Work out the finished part from the listing and answer in its coordinate system (mm). A direction names the side the tool comes from. Give positions to 0.01 mm unless a question says otherwise; leave off trailing zeros. Write each loop counter-clockwise with the first axis right and the second up, starting at its lowest first coordinate (ties: lowest second). Pieces come first, ordered by that corner, then holes. Notation, with made-up numbers: (15, 55.5) -> (22, 55.5) arc R31 ccw to (22, 82.5) -> close; hole circle Ø10 at (-30.75, -22). An arc over 180 degrees is marked (long way). Write item = value, one per line. Start each with the question number.
Autodesk Inventor part; units mm, degrees
ref_plane "YZ Plane" through (0, 0, 0) normal (1, 0, 0) x (0, 1, 0)
ref_plane "XZ Plane" through (0, 0, 0) normal (0, 1, 0) x (-1, 0, 0)
ref_plane "XY Plane" through (0, 0, 0) normal (0, 0, 1) x (1, 0, 0)
sketch "Sketch1" plane through (0, 0, 0) normal (0, 0, 1) x (1, 0, 0)
  circle A0 centre (0, 0) radius 1.778
  circle A1 centre (0, 0) radius 32.512
  circle A2 centre (0, 0) radius 26.162
  circle A3 centre (0, 0) radius 6.858
  line L0 (-3.048, 6.1434) -> (-6.8485, 25.2497)
  line L1 (3.048, 6.1434) -> (6.8485, 25.2497)
  arc A4 (6.8485, 25.2497) -> (-6.8485, 25.2497) centre (0, 0) ccw construction
  line L2 (-6.7846, -1.0004) -> (-26.1302, 1.2893)
  circle A5 centre (0, 0) radius 26.162
  line L3 (-4.9009, 4.7972) -> (-21.8976, 14.3159)
  circle A6 centre (0, 0) radius 6.858
  line L4 (-1.1451, -6.7617) -> (-9.3009, -24.4529)
  circle A7 centre (0, 0) radius 26.162
  line L5 (-6.0769, -3.1786) -> (-20.3819, -16.402)
  circle A8 centre (0, 0) radius 6.858
  line L6 (6.0769, -3.1786) -> (20.3819, -16.402)
  circle A9 centre (0, 0) radius 26.162
  line L7 (1.1451, -6.7617) -> (9.3009, -24.4529)
  circle A10 centre (0, 0) radius 6.858
  line L8 (4.9009, 4.7972) -> (21.8976, 14.3159)
  circle A11 centre (0, 0) radius 26.162
  line L9 (6.7846, -1.0004) -> (26.1302, 1.2893)
  circle A12 centre (0, 0) radius 6.858
  dimension "d1" = 65.024
  dimension "d2" = 3.556
  dimension "d3" = 13.716
  dimension "d4" = 6.35
  dimension "d5" = 22.5
  dimension "d7" = 3.048
  dimension "d10" = 360
extrude "Extrusion1" add sketch "Sketch1" along normal blind 26.924 contours A1 | A3
extrude "Extrusion2" add sketch "Sketch1" along normal blind 21.59 contours A0
extrude "Extrusion3" add sketch "Sketch1" along normal blind 5.334 contours L9 A3 L8 A2 | A2 L7 A3 L6 | L1 A3 L0 A2 | A2 L5 A3 L4 | L3 A3 L2 A2
fillet "Fillet1" radius 3.175 2 edges at (-32.512, 0, 26.924) (-32.512, 0, 0)
properties part number "OGWheel" material "ABS Plastic"
(1) Find the intervals of material crossed by line 1 along Y through (x, z) = (1, 9.5); line 2 along Y through (x, z) = (0, 13); line 3 along Y through (x, z) = (0, 25.6), in increasing order.
(2) For faces 1 (the flat face through (5.166, -15.483, 2.63)), 2 (the flat face through (1.4, -1.4, 26.924)), 3 (the cylindrical face through (6.54, -2.06, 16.27)), determine the directions among +Z, -Z, +X, -X, +Y, -Y from which every point of the face is accessible in a straight line to the end or side of a thin tool.
(3) Each of these flat-tipped pins is pushed along its axis until it touches: pin 1 (7.5 mm diameter, centred on x = 19.5, y = 5.5, fed in from +Z); pin 2 (10 mm diameter, centred on y = -16.5, z = 13.5, fed in from -X); pin 3 (2 mm diameter, centred on x = -22, y = 24, fed in from +Z). Where does it stop, or does it pass through?
(4) A cutting plane is placed at A-A, the plane x = 0. Write down the section's boundary in (y, z) (3 decimals).
(5) A cutting plane is placed at D-D, the plane x = -12.5. State how many separate pieces and enclosed holes the cut face has, then the cut area to 3 significant figures.
(6) A cutting plane is placed at C-C, the plane y = 0. Write down the section's boundary in (x, z) (3 decimals).
(7) A cutting plane is placed at B-B, the plane z = 16.5. Write down the section's boundary in (x, y), then the cut area to 3 significant figures.
(8) Determine the mould class of faces 4 (the flat face through (-4.92, 15.56, 2.63)), 5 (the flat face through (-26.2, -4.2, 26.924)) for opening direction Y: pulls with the +Y half, pulls with the -Y half, needs draft (parallel to the pull), parting line crosses it, or undercut.
Results list:
q1.line_1 = -32.5 to -26.14, -6.78 to 6.78, 26.14 to 32.5
q1.line_2 = -32.51 to -26.16, -6.86 to 6.86, 26.16 to 32.51
q1.line_3 = -31.92 to -26.16, -6.86 to -1.78, 1.78 to 6.86, 26.16 to 31.92
q2.face_1 = +Z, -Z
q2.face_2 = +Z, +X, -X, +Y, -Y
q2.face_3 = +Z
q3.pin_1 = 5.33
q3.pin_2 = -30.41
q3.pin_3 = 26.02
q4.outline = (-32.512, 3.175) arc R3.175 ccw to (-29.337, 0) -> (-26.162, 0) -> (-26.162, 26.924) -> (-29.337, 26.924) arc R3.175 ccw to (-32.512, 23.749) -> close; (-6.858, 0) -> (29.337, 0) arc R3.175 ccw to (32.512, 3.175) -> (32.512, 23.749) arc R3.175 ccw to (29.337, 26.924) -> (26.162, 26.924) -> (26.162, 5.334) -> (6.858, 5.334) -> (6.858, 26.924) -> (1.778, 26.924) -> (1.778, 21.59) -> (-1.778, 21.59) -> (-1.778, 26.924) -> (-6.858, 26.924) -> close
q5.separate_pieces = 3
q5.enclosed_holes = 0
q5.area = 493 mm²
q6.outline = (-32.512, 3.175) arc R3.175 ccw to (-29.337, 0) -> (-26.162, 0) -> (-26.162, 26.924) -> (-29.337, 26.924) arc R3.175 ccw to (-32.512, 23.749) -> close; (-15.237, 0) -> (15.237, 0) -> (15.237, 5.334) -> (6.858, 5.334) -> (6.858, 26.924) -> (1.778, 26.924) -> (1.778, 21.59) -> (-1.778, 21.59) -> (-1.778, 26.924) -> (-6.858, 26.924) -> (-6.858, 5.334) -> (-15.237, 5.334) -> close; (26.162, 0) -> (29.337, 0) arc R3.175 ccw to (32.512, 3.175) -> (32.512, 23.749) arc R3.175 ccw to (29.337, 26.924) -> (26.162, 26.924) -> close
q7.outline = circle Ø65.02 at (0, 0); circle Ø13.72 at (0, 0); hole circle Ø52.32 at (0, 0)
q7.area = 1,320 mm²
q8.face_4 = undercut
q8.face_5 = needs draft
